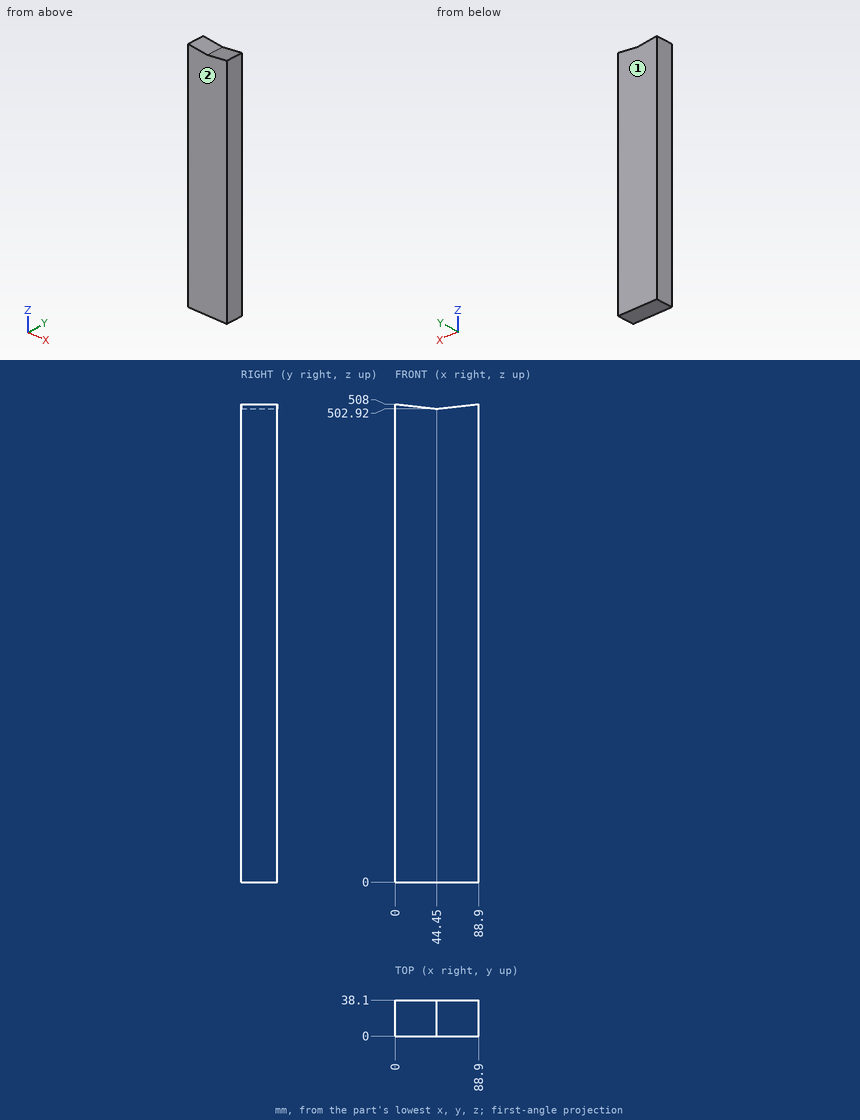
Verification items for this drawing (mm, ordinates from the low corner). Give positions to 0.01 mm unless a question says otherwise; leave off trailing zeros.
1) Material ranges on L1, parallel to Z at x = 79.5, y = 4; L2, parallel to Z at x = 44, y = 7.5, recorded low to high.
2) Gauge pin test, flat ends, axial feed: pin 1 (3 mm diameter, centred on x = 39, y = 5, fed in from -Z); pin 2 (6 mm diameter, centred on x = 13, y = 21, fed in from +Z). Record the tip position at first contact, or that the pin passes through.
3) Release check for a two-part mould opening along Y. For the marked faces 1 and 2 record: pulls with the +Y half, pulls with the -Y half, needs draft (parallel to the pull), parting line crosses it, or undercut.
Computed:
1. L1: z = 0 to 506.93
1. L2: z = 0 to 502.97
2. pin 1: stops at z = 0
2. pin 2: stops at z = 506.86
3. face 1: pulls with the +Y half
3. face 2: pulls with the -Y half
